Can you work these out from the drawing? Everything is in mm from the part's minimum corner. Coordinates: 2 decimals unless noted, no trailing zeros. Order: outer loops, then holes, each group sorted by start corner. A loop starts at its lowest first (then second) coordinate and runs counter-clockwise, first axis right, second up. Notation, with made-up numbers: (64.25, 3.5) -> (121.25, 3.5) arc R22 cw to (121.25, 24.5) -> close; hole circle Ø8 at (38, 86.5). An arc over 180 degrees is marked (long way). Return JSON: item names as keys, results as strings. Group by question number.
1) If we section it at C-C, the plane z = 16.5: Please give me the cut outline in (x, y), then the cut area to 3 significant figures.
2) If I drill on probe 1 along X at (y, z) = (24.5, 23); probe 2 along Z at (x, y) = (26.5, 36.5), over which ranges is the centre line in solid material (lowest first)? Write a range as from..to.
3) If we section it at A-A, the plane x = 24.5: Please give me the cut outline in (y, z).
4) For pin 1 (1 mm diameter, centred on y = 43, z = 45.5, fed in from -X); pin 2 (3 mm diameter, centred on x = 30.5, z = 33.5, fed in from -Y); pin 3 (22.5 mm diameter, centred on x = 15.5, y = 19, fed in from +Z), each with a flat end and sliding along its axis, tell me the tip position at first contact or that it passes through.
5) Thinking about a two-plate mould opening in X: for the marked faces 1, 2 and 3, which applies, +X half, -X half, draft (parallel to the pull), parting line (faces both ways), or undercut?
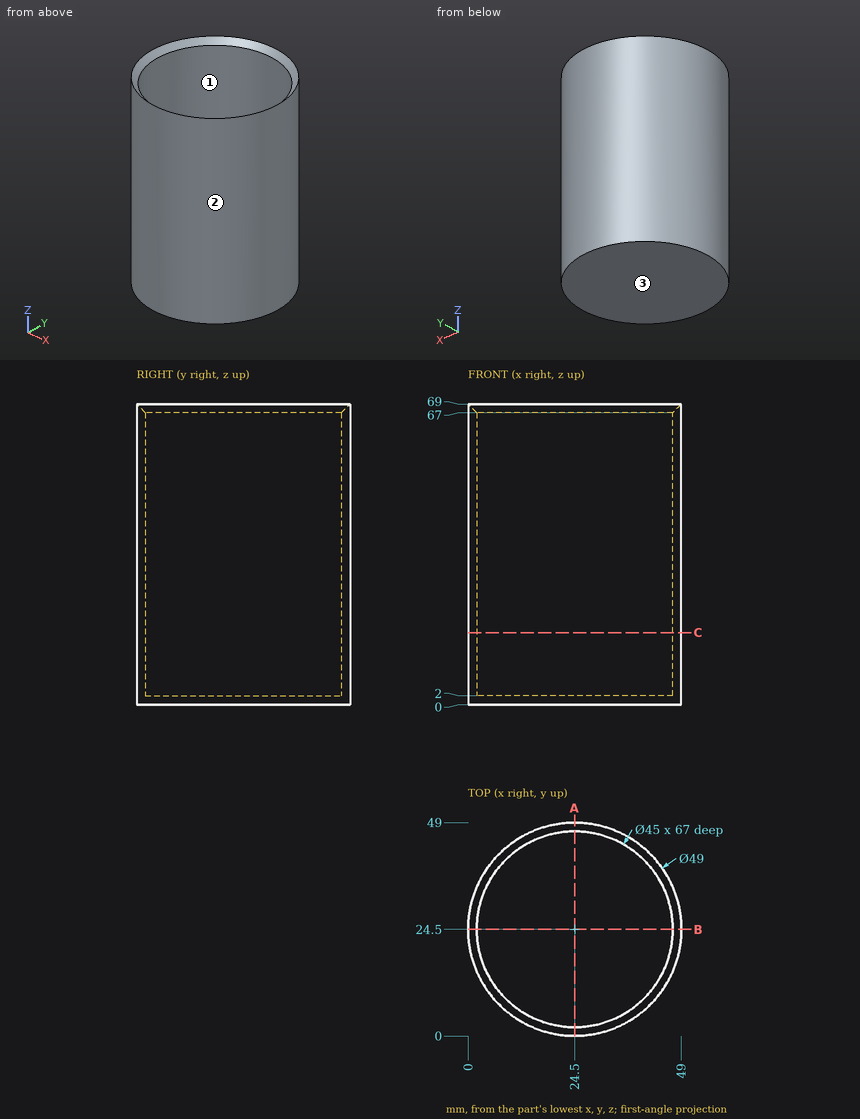
Result sheet:
{
 "1": {"outline": "circle Ø49 at (24.5, 24.5); hole circle Ø45 at (24.5, 24.5)", "area": "295 mm2"},
 "2": {"probe 1": "x = 0..2, 47..49", "probe 2": "z = 0..2"},
 "3": {"outline": "(0, 0) -> (49, 0) -> (49, 69) -> (47, 67) -> (47, 2) -> (2, 2) -> (2, 67) -> (0, 69) -> close"},
 "4": {"pin 1": "stops at x = 7.88", "pin 2": "stops at y = 0.42", "pin 3": "stops at z = 2"},
 "5": {"face 1": "undercut", "face 2": "parting line", "face 3": "draft"}
}
